```python
from build123d import *

# Parameters (mm, degrees)
F0_W     = 71
F0_H     = 15
F1_DEPTH = 4
F0_H_2   = 111
F2_DEPTH = 1
F3_R     = 5


with BuildPart() as f1:
    # F0 (on Front) → F1 (new body)
    with BuildSketch(Plane.XZ):
        with Locations((0, 63)):
            Rectangle(F0_W, F0_H)
        with Locations((0, -63)):
            Rectangle(F0_W, F0_H)
    extrude(amount=F1_DEPTH)

    # F0 (on Front) → F2 (join)
    with BuildSketch(Plane.XZ):
        Rectangle(F0_W, F0_H_2)
    extrude(amount=F2_DEPTH)

    # F3
    f3_edges = [f1.edges().sort_by_distance(p)[0] for p in [
        (-35.5, -2, 70.5),
        (35.5, -2, 70.5),
        (35.5, -2, -70.5),
        (-35.5, -2, -70.5),
    ]]
    fillet(f3_edges, radius=F3_R)


solid = f1.part
```
Here's how the part is built. I have some questions about the finished solid (model axes, mm). A direction names the side the tool comes from. Coordinates: 2 decimals unless noted, no trailing zeros. Order: outer loops, then holes, each group sorted by start corner. A loop starts at its lowest first (then second) coordinate and runs counter-clockwise, first axis right, second up. Notation, with made-up numbers: (9.25, 35.25) -> (53.25, 35.25) arc R19 cw to (53.25, 42.25) -> close; hole circle Ø4 at (-19.75, 88.5). An arc over 180 degrees is marked (long way). Return JSON: item names as keys, results as strings.
1) If we section it at C-C on z = 47: List the corners of the cut face in (x, y) for me.
Conclusion:
{"outline": "(-35.5, -1) -> (35.5, -1) -> (35.5, 0) -> (-35.5, 0) -> close"}
2) On a 3-axis mill with a long thin cutter (end or side, diameter ignored), from which of +Z, -Z, +X, -X, +Y, -Y can I reach the whole of each face in a straight line? I mean faces 4 (the flat face through (0, -1, 1)), 5 (the cylindrical face through (-34.07, -2.03, -69)). Say none if no direction works.
Conclusion:
{"face 4": "+X, -X, -Y", "face 5": "-Z, -X, +Y, -Y"}
3) If we section it at B-B on x = 13.5: List the corners of the cut face in (y, z) for me, plus the area to 3 significant figures.
Conclusion:
{"outline": "(-4, -70.5) -> (0, -70.5) -> (0, 70.5) -> (-4, 70.5) -> (-4, 55.5) -> (-1, 55.5) -> (-1, -55.5) -> (-4, -55.5) -> close", "area": "231 mm²"}
4) Thinking about a two-plate mould opening in Z: for faces 1 (the flat face through (0, -2, -55.5)), 2 (the flat face through (0, 0, 1)), 3 (the flat face through (0, -2, -70.5)), which applies, +Z half, -Z half, draft (parallel to the pull), parting line (faces both ways), or undercut?
Conclusion:
{"face 1": "undercut", "face 2": "draft", "face 3": "-Z half"}
5) If I drill on probe 1 along Z at (x, y) = (-8, -3.1); probe 2 along Y at (x, z) = (15.5, 19); probe 3 along Z at (x, y) = (-31.5, -0.6), over which ranges is the centre line in solid material (lowest first)?
Conclusion:
{"probe 1": "z = -70.5 to -55.5, 55.5 to 70.5", "probe 2": "y = -1 to 0", "probe 3": "z = -70.4 to 70.4"}
6) If we section it at A-A on y = -3.1: List the corners of the cut face in (x, z) for me.
Conclusion:
{"outline": "(-35.5, -65.5) arc R5 ccw to (-30.5, -70.5) -> (30.5, -70.5) arc R5 ccw to (35.5, -65.5) -> (35.5, -55.5) -> (-35.5, -55.5) -> close; (-35.5, 55.5) -> (35.5, 55.5) -> (35.5, 65.5) arc R5 ccw to (30.5, 70.5) -> (-30.5, 70.5) arc R5 ccw to (-35.5, 65.5) -> close"}
7) I'm going to push flat-ended pins straight in: P1, Ø5, axis at x = 22, z = 34, coming from the +Y side; P2, Ø12, axis at x = -12, z = -20, coming from the -Y side. Where does each tip first touch, or does it pass through?
Conclusion:
{"P1": "stops at y = 0", "P2": "stops at y = -1"}
